```python
from build123d import *

# Parameters (mm, degrees)
F0_W     = 12.954
F0_H     = 12.192
F0_R     = 3.175
F0_H_2   = 1.5748
F1_DEPTH = 1.524
F2_DEPTH = 12.192
F3_SIZE  = 1.27
F5_W     = 16.256
F5_H     = 12.954
F5_R     = 2.0955
F6_DEPTH = 1.5748
F7_R     = 1.5494


# Not quite as in the source:
# - a feature names something its author has since deleted; it is built from what else it names


with BuildPart() as f1:
    # F0 (on Right) → F1 (new body)
    with BuildSketch(Plane.YZ):
        with BuildLine():
            ThreePointArc((6.477, 6.096), (0, 8.636), (-6.477, 6.096))
            Line((-6.477, 6.096), (6.477, 6.096))
        make_face()
        Rectangle(F0_W, F0_H)
        with Locations((0, 1.651)):
            Circle(F0_R, mode=Mode.SUBTRACT)
        with Locations((0, -6.8834)):
            Rectangle(F0_W, F0_H_2)
        with Locations((0, 1.651)):
            Circle(F0_R)
    extrude(amount=-F1_DEPTH)

    # F0 (on Right) → F2 (join)
    with BuildSketch(Plane.YZ):
        with Locations((0, 1.651)):
            Circle(F0_R)
    extrude(amount=-F2_DEPTH)

    # F3
    f3_edges = [f1.edges().sort_by_distance(p)[0] for p in [
        (-12.192, -3.175, 1.651),
    ]]
    chamfer(f3_edges, length=F3_SIZE)

    # F5 (on offset) → F6 (join)
    with BuildSketch(Plane(origin=(0, 0, -7.6708), x_dir=(1, 0, 0), z_dir=(0, 0, -1))):
        with Locations((8.128, 0)):
            Rectangle(F5_W, F5_H)
        with Locations((9.5885, 0)):
            Circle(F5_R, mode=Mode.SUBTRACT)
        with BuildLine():
            Line((16.256, 6.477), (16.256, -6.477))
            ThreePointArc((16.256, -6.477), (18.542, 0), (16.256, 6.477))
        make_face()
    extrude(amount=-F6_DEPTH)

    # F7
    f7_edges = [f1.edges().sort_by_distance(p)[0] for p in [
        (-1.524, 0, -7.6708),
    ]]
    fillet(f7_edges, radius=F7_R)


solid = f1.part
```
CAD build for the part. Positions are in the model's coordinates, mm. A direction names the side the tool comes from. Coordinates: 2 decimals unless noted, no trailing zeros. Order: outer loops, then holes, each group sorted by start corner. A loop starts at its lowest first (then second) coordinate and runs counter-clockwise, first axis right, second up. Notation, with made-up numbers: M 66.25,-30.75 L 88.25,-30.75 A14 cw 88.25,-17.75 Z; hole C -24.5,23 d11. An arc over 180 degrees is marked long. Answer as CSV lines item,"result".
1) Cut at A-A (y = 0). List the corners of the cut face in (x, z), then the cut area to 3 significant figures.
Verdict:
outline,"M -12.19,-0.25 L -10.92,-1.52 L -1.52,-1.52 L -1.52,-6.12 A1.55 ccw 0.03,-7.67 L 7.49,-7.67 L 7.49,-6.1 L 0,-6.1 L 0,8.64 L -1.52,8.64 L -1.52,4.83 L -10.92,4.83 L -12.19,3.56 Z; M 11.68,-7.67 L 18.54,-7.67 L 18.54,-6.1 L 11.68,-6.1 Z"
area,"113 mm2"
2) Cut at D-D (x = 5). List the corners of the cut face in (y, z).
Verdict:
outline,"M -6.48,-7.67 L 6.48,-7.67 L 6.48,-6.1 L -6.48,-6.1 Z"
3) Drill centre lines: L1, parallel to Z at x = 2, y = 0.5; L2, parallel to X at y = 1, z = -7; L3, parallel to X at y = -2.25, z = -1.75. Where is each one in solid material? Low to high. Write a range as from..to.
Verdict:
L1,"-7.67..-6.1"
L2,"-1.25..7.75, 11.43..18.49"
L3,"-1.52..0"
4) Flat gauge pins, fed straight in: P1, Ø4, axis at y = 4, z = -5.5, coming from the -X side; P2, Ø1, axis at x = 4.5, z = -6, coming from the +Y side; P3, Ø1.5, axis at x = -3.5, y = -0.5, coming from the -Z side; P4, Ø5, axis at x = 9.59, y = 0, coming from the +Z side. Where does each tip first touch, or does it go through?
Verdict:
P1,"x = -1.52"
P2,"y = 6.48"
P3,"z = -1.52"
P4,"z = -6.1"
5) Cut at C-C (z = -2.5). List the corners of the cut face in (x, y), then the cut area to 3 significant figures.
Verdict:
outline,"M -1.52,-6.48 L 0,-6.48 L 0,6.48 L -1.52,6.48 Z"
area,"19.7 mm2"
6) Cut at B-B (y = 4.25). List the corners of the cut face in (x, z).
Verdict:
outline,"M -1.52,-6.12 A1.55 ccw 0.03,-7.67 L 17.63,-7.67 L 17.63,-6.1 L 0,-6.1 L 0,7.64 L -1.52,7.64 Z"
7) Mould opens along X. For faces 1 (the cylindrical face through (-6.2, -0.4, 4.8)), 2 (the cylindrical face through (-1.082, 0.091, -7.205)), 3 (the flat face through (0, 0, 1)), 4 (the cylindrical face through (11.524, 0.803, -6.894)) say: released by +X, released by -X, zero draft, split by the parting line, or undercut.
Verdict:
face 1,"zero draft"
face 2,"released by -X"
face 3,"released by +X"
face 4,"undercut"
8) 3-axis set-ups, long thin cutter, end or side, ignore diameter. For faces 5 (the flat face through (7, 0, -6.096)), 6 (the flat face through (-1.524, 0, -2)), 7 (the flat face through (4, 6.477, -6.4)): which of +Z, -Z, +X, -X, +Y, -Y reach the whole face in a straight line?
Verdict:
face 5,"+Z, +X, +Y, -Y"
face 6,"-X"
face 7,"+Z, -Z, +X, -X, +Y"
